Geometry check sheet. Reference: the model listing, model coordinates, mm. A direction names the side the tool comes from. Give positions to 0.01 mm unless a question says otherwise; leave off trailing zeros. Write each loop counter-clockwise with the first axis right and the second up, starting at its lowest first coordinate (ties: lowest second). Pieces come first, ordered by that corner, then holes. Notation, with made-up numbers: (-17, -28) - (16, -28) arc R27 cw to (16, -1) - close; hole circle Ø4 at (38, 66.25). An arc over 180 degrees is marked (long way). Use a Markdown table: item, result.
```python
from build123d import *

# Parameters (mm, degrees)
SKETCH1_W           = 50
SKETCH1_H           = 70
BOSS_EXTRUDE1_DEPTH = 40
SKETCH3_R           = 15
BOSS_EXTRUDE3_DEPTH = 100
BOSS_EXTRUDE4_START = 120
SKETCH4_R           = 15
BOSS_EXTRUDE4_DEPTH = 120


with BuildPart() as part:
    # Sketch1 → Boss-Extrude1 (new body)
    with BuildSketch(Plane.XY):
        with Locations((-25, 35)):
            Rectangle(SKETCH1_W, SKETCH1_H)
    extrude(amount=BOSS_EXTRUDE1_DEPTH)

    # Sketch3 → Boss-Extrude3 (add)
    with BuildSketch(Plane.ZY.offset(50)):
        with Locations((20, 35)):
            Circle(SKETCH3_R)
    extrude(amount=BOSS_EXTRUDE3_DEPTH)

    # Sketch4 → Boss-Extrude4 (add)
    with BuildSketch(Plane(origin=(0, 0, 0), x_dir=(0, 0, -1), z_dir=(1, 0, 0)).offset(BOSS_EXTRUDE4_START)):
        with Locations(Location((-20, 35, 0), (0, 0, 180))):
            Circle(SKETCH4_R)
    extrude(amount=-BOSS_EXTRUDE4_DEPTH)


solid = part.part
```
1) Section check D-D on y = 56. Record the boundary of the cut face in (x, z).
Working result:
| item | result |
|---|---|
| outline | (-50, 0) - (0, 0) - (0, 40) - (-50, 40) - close |
2) Set-up check for faces 1 (the cylindrical face through (60.84, 24.862, 8.944)), 2 (the cylindrical face through (-99.3, 45.138, 8.944)), 3 (the flat face through (-25, 35, 40)): record each of +Z, -Z, +X, -X, +Y, -Y from which the full face is reachable in a straight line by a thin tool's end or side.
Working result:
| item | result |
|---|---|
| face 1 | +X |
| face 2 | -X |
| face 3 | +Z, +X, -X, +Y, -Y |
3) Material ranges on L1, parallel to X at y = 8.5, z = 5.5; L2, parallel to Z at x = 46, y = 35; L3, parallel to Z at x = 104, y = 44, recorded low to high. Write a range as from..to.
Working result:
| item | result |
|---|---|
| L1 | x = -50..0 |
| L2 | z = 5..35 |
| L3 | z = 8..32 |
4) Section check B-B on y = 35. Record the boundary of the cut face in (x, z), then the cut area to 3 significant figures.
Working result:
| item | result |
|---|---|
| outline | (-150, 5) - (-50, 5) - (-50, 0) - (0, 0) - (0, 5) - (120, 5) - (120, 35) - (0, 35) - (0, 40) - (-50, 40) - (-50, 35) - (-150, 35) - close |
| area | 8,600 mm² |
5) Section check C-C on x = 65. Record the boundary of the cut face in (y, z).
Working result:
| item | result |
|---|---|
| outline | circle Ø30 at (35, 20) |
6) Depth check by flat-ended pin: P1, Ø8, axis at x = 37, z = 18.5, coming from the -Y side; P2, Ø1, axis at x = -54.5, y = 48.5, coming from the +Z side; P3, Ø4, axis at x = 63, z = 19.5, coming from the +Y side. Enter the tip coordinate at first touch or a pass-through.
Working result:
| item | result |
|---|---|
| P1 | stops at y = 20 |
| P2 | stops at z = 27.48 |
| P3 | stops at y = 50 |
7) Section check A-A on z = 20. Record the boundary of the cut face in (x, y), then the cut area to 3 significant figures.
Working result:
| item | result |
|---|---|
| outline | (-150, 20) - (-50, 20) - (-50, 0) - (0, 0) - (0, 20) - (120, 20) - (120, 50) - (0, 50) - (0, 70) - (-50, 70) - (-50, 50) - (-150, 50) - close |
| area | 10,100 mm² |
